Read the model definition and answer for the solid it produces. Units are mm, in the model's axes. Round coordinates to 2 decimals unless told otherwise and drop trailing zeros. Loops run counter-clockwise (first coordinate to the right, second up) from the corner with the lowest first, then second, coordinate; pieces in that order, holes last. Notation, with made-up numbers: (-34, 37) - (-14, 37) arc R26 cw to (-14, 55) - close; hole circle Ø10 at (50, -36.5). An arc over 180 degrees is marked (long way). Answer as CSV lines item,"result".
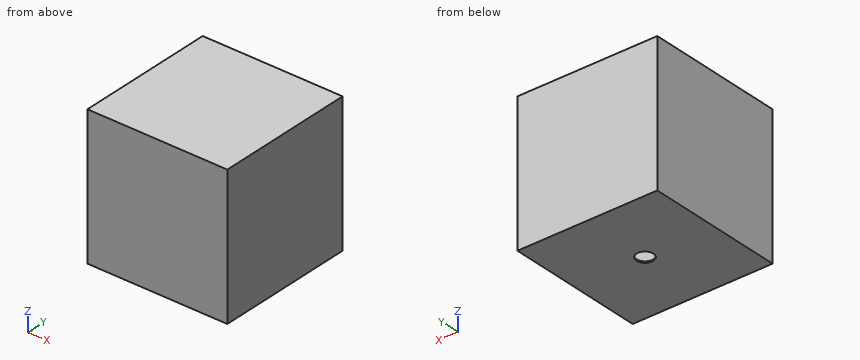
```python
from build123d import *

# Parameters (mm, degrees)
ESQUISSE1_W             = 50
ESQUISSE1_H             = 50
BOSS_EXTRU_1_DEPTH      = 50
COQUE2_T                = -0.5
ESQUISSE2_R             = 3
ENL_V_MAT_EXTRU_1_DEPTH = 5
ESQUISSE3_W             = 50
ESQUISSE3_H             = 50
BOSS_EXTRU_2_DEPTH      = 1


with BuildPart() as part:
    # Esquisse1 → Boss.-Extru.1 (new body)
    with BuildSketch(Plane.XY):
        Rectangle(ESQUISSE1_W, ESQUISSE1_H)
    extrude(amount=BOSS_EXTRU_1_DEPTH)

    # Coque2
    coque2_openings = [part.faces().sort_by_distance(p)[0] for p in [
        (0, 0, 50),
    ]]
    offset(amount=COQUE2_T, openings=coque2_openings, kind=Kind.INTERSECTION)

    # Esquisse2 → Enl_v. mat.-Extru.1 (cut)
    with BuildSketch(Plane(origin=(0, 0, 0), x_dir=(-1, 0, 0), z_dir=(0, 0, -1))):
        Circle(ESQUISSE2_R)
    extrude(amount=-ENL_V_MAT_EXTRU_1_DEPTH, mode=Mode.SUBTRACT)

    # Esquisse3 → Boss.-Extru.2 (add)
    with BuildSketch(Plane.XY.offset(50)):
        Rectangle(ESQUISSE3_W, ESQUISSE3_H)
    extrude(amount=-BOSS_EXTRU_2_DEPTH)


solid = part.part
```
1) This flat-tipped pin is pushed along its axis until it touches: P1, Ø14.5, axis at x = 5.5, y = 0.5, coming from the -Z side. Where does it stop, or does it pass through?
Entries:
P1,"stops at z = 0"
2) Find the intervals of material crossed by line 1 (Y direction, x = 0, z = 0.25); line 2 (Y direction, x = 3.5, z = 17); line 3 (Z direction, x = 21, y = -6), in increasing order.
Entries:
line 1,"y = -25 to -3, 3 to 25"
line 2,"y = -25 to -24.5, 24.5 to 25"
line 3,"z = 0 to 0.5, 49 to 50"
3) A cutting plane is placed at C-C, the plane y = 0. Determine the outline of the cut face in (x, z), plus the area to 4 significant figures.
Entries:
outline,"(-25, 0) - (-3, 0) - (-3, 0.5) - (-24.5, 0.5) - (-24.5, 49) - (24.5, 49) - (24.5, 0.5) - (3, 0.5) - (3, 0) - (25, 0) - (25, 50) - (-25, 50) - close"
area,"120.5 mm^2"
4) A cutting plane is placed at A-A, the plane x = 21. Determine the outline of the cut face in (y, z), plus the area to 4 significant figures.
Entries:
outline,"(-25, 0) - (25, 0) - (25, 50) - (-25, 50) - close; hole (-24.5, 0.5) - (24.5, 0.5) - (24.5, 49) - (-24.5, 49) - close"
area,"123.5 mm^2"
